Input: dimensioned drawing with shaded views. Units: mm. Origin: part minimum x, y, z. Round coordinates to 2 decimals unless told otherwise and drop trailing zeros. Write each loop counter-clockwise with the first axis right and the second up, starting at its lowest first coordinate (ties: lowest second). Pieces come first, ordered by that corner, then holes. Notation, with made-up numbers: M 10,61.25 L 36,61.25 A19 ccw 36,78.25 Z; hole C 40,1.25 d4. An arc over 180 degrees is marked long. Use one line per item in the form item = value. Start each with the question number.
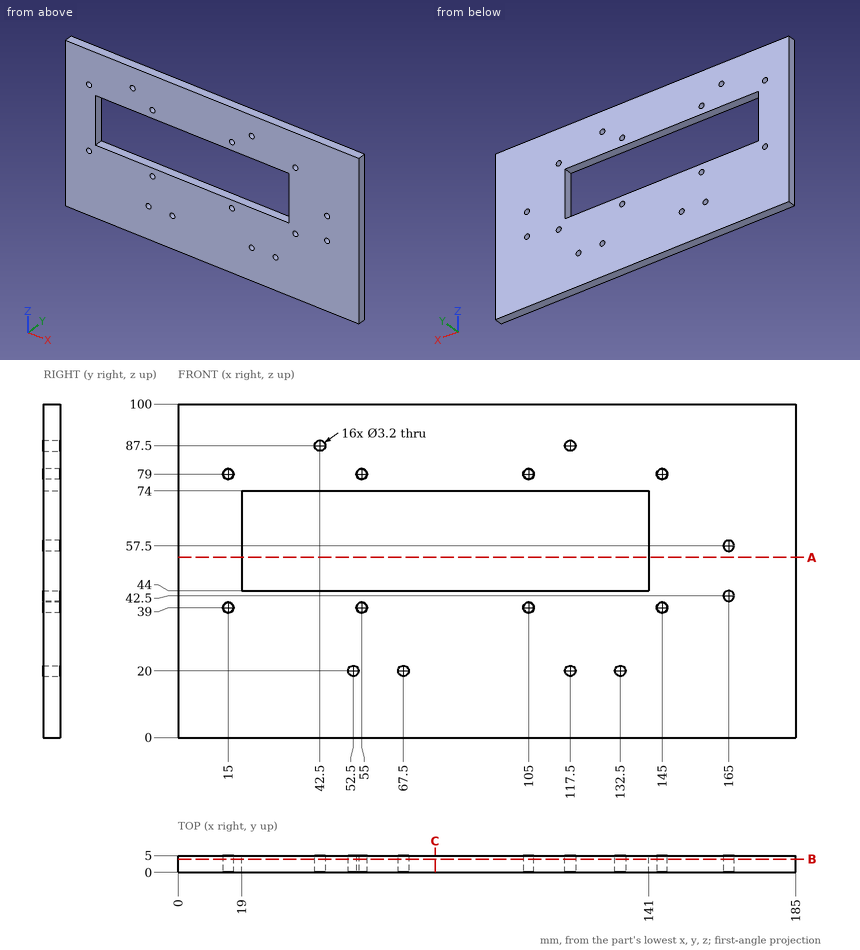
1. Section query B-B (y = 3.95). Give the number of separate pieces and of enclosed holes in the cut face, then the cut area to 3 significant figures.
2. Section query A-A (z = 54). Return loops of the section in (x, y), then the cut area to 3 significant figures.
3. Ray query, probe 1 along Z at (x, y) = (42.5, 3.25); probe 2 along Z at (x, y) = (15, 2); probe 3 along X at (y, z) = (1.85, 79). Return the intervals inside material, ascending.
4. Section query C-C (x = 77). Return loops of the section in (y, z), then the cut area to 3 significant figures.
Checks:
q1.separate_pieces = 1
q1.enclosed_holes = 17
q1.area = 14,700 mm^2
q2.outline = M 0,0 L 19,0 L 19,5 L 0,5 Z; M 141,0 L 185,0 L 185,5 L 141,5 Z
q2.area = 315 mm^2
q3.probe_1 = 0 to 44, 74 to 85.9, 89.1 to 100
q3.probe_2 = 0 to 37.4, 40.6 to 77.4, 80.6 to 100
q3.probe_3 = 0 to 13.4, 16.6 to 53.4, 56.6 to 103.4, 106.6 to 143.4, 146.6 to 185
q4.outline = M 0,0 L 5,0 L 5,44 L 0,44 Z; M 0,74 L 5,74 L 5,100 L 0,100 Z
q4.area = 350 mm^2
